```python
from build123d import *

# Parameters (mm, degrees)
BOSS_EXTRU_1_DEPTH      = 8
CONG_1_R                = 7.5
ENL_V_MAT_EXTRU_1_REACH = 29.299
ESQUISSE2_R             = 2
ESQUISSE3_R             = 7
ESQUISSE3_R_2           = 4
BOSS_EXTRU_2_DEPTH      = 8


with BuildPart() as part:
    # Esquisse1 → Boss.-Extru.1 (new body)
    with BuildSketch(Plane(origin=(0, 0, 0), x_dir=(1, 0, 0), z_dir=(0, 1, 0))):
        Polygon((0, -7.5), (25, -7.5), (25, 7.5), (0, 7.5), (-25, 7.5), (-25, -7.5), align=None)
    extrude(amount=BOSS_EXTRU_1_DEPTH)

    # Congé1
    cong_1_edges = [part.edges().sort_by_distance(p)[0] for p in [
        (-25, 4, 7.5),
        (-25, 4, -7.5),
        (25, 4, -7.5),
        (25, 4, 7.5),
    ]]
    fillet(cong_1_edges, radius=CONG_1_R - 0.0001)  # a hair under: the kernel refuses the full size

    # Esquisse2 → Enlèv. mat.-Extru.1 (cut, up to next)
    with BuildSketch(Plane(origin=(0, 8, 0), x_dir=(1, 0, 0), z_dir=(0, 1, 0)), mode=Mode.PRIVATE) as enl_v_mat_extru_1_sk1:
        with Locations(Location((-15, 0, 0), (0, 0, 270))):
            Circle(ESQUISSE2_R)
    enl_v_mat_extru_1_tool1 = extrude(enl_v_mat_extru_1_sk1.sketch, amount=-ENL_V_MAT_EXTRU_1_REACH, mode=Mode.PRIVATE) & part.part
    # Esquisse2 → Enlèv. mat.-Extru.1 (cut, up to next)
    with BuildSketch(Plane(origin=(0, 8, 0), x_dir=(1, 0, 0), z_dir=(0, 1, 0)), mode=Mode.PRIVATE) as enl_v_mat_extru_1_sk2:
        with Locations(Location((15, 0, 0), (0, 0, 270))):
            Circle(ESQUISSE2_R)
    enl_v_mat_extru_1_tool2 = extrude(enl_v_mat_extru_1_sk2.sketch, amount=-ENL_V_MAT_EXTRU_1_REACH, mode=Mode.PRIVATE) & part.part
    add(enl_v_mat_extru_1_tool1.solids().sort_by_distance((-15, 8, 0))[0], mode=Mode.SUBTRACT)
    add(enl_v_mat_extru_1_tool2.solids().sort_by_distance((15, 8, 0))[0], mode=Mode.SUBTRACT)

    # Esquisse3 → Boss.-Extru.2 (add)
    with BuildSketch(Plane(origin=(0, 8, 0), x_dir=(1, 0, 0), z_dir=(0, 1, 0))):
        with Locations(Location((0, 0, 0), (0, 0, 90))):
            Circle(ESQUISSE3_R)
        with Locations(Location((0, 0, 0), (0, 0, 270))):
            Circle(ESQUISSE3_R_2, mode=Mode.SUBTRACT)
    extrude(amount=BOSS_EXTRU_2_DEPTH)


solid = part.part
```
Could you check a few things on this model? Use its own coordinates, in mm. A direction names the side the tool comes from. Round coordinates to 2 decimals unless told otherwise and drop trailing zeros. Write each loop counter-clockwise with the first axis right and the second up, starting at its lowest first coordinate (ties: lowest second). Pieces come first, ordered by that corner, then holes. Notation, with made-up numbers: M 31,39 L 58,39 A27 ccw 58,62 Z; hole C -24.5,54.5 d8. An arc over 180 degrees is marked long. Answer in a Markdown table with one row per item. Add a question column.
Q1. Imagine slicing it at C-C (z = 1). Please give me the cut outline in (x, y), then the cut area to 3 significant figures.
Q2. Imagine slicing it at B-B (y = 2.25). Give the number of separate pieces and of enclosed holes in the cut face, then the cut area to 3 significant figures.
Q3. If I drill on line 1 (X direction, y = 4.25, z = 0); line 2 (X direction, y = 11.25, z = 0); line 3 (Y direction, x = -11, z = 4), over which ranges is the centre line in solid material (lowest first)? Write a range as from..to.
Q4. Imagine slicing it at A-A (x = 15). Please give me the cut outline in (y, z).
Q5. If we mould it in two halves opening along X, with no side actions, what happens to faces 1 (the cylindrical face through (-22.745, 4.056, -5.361)), 2 (the flat face through (0, 0, 0)), 3 (the cylindrical face through (-3.905, 11.944, -0.867)), 4 (the flat face through (0, 8, 0))? For each: +X half, -X half, draft (parallel to the pull), parting line (faces both ways), or undercut.
Q6. Imagine slicing it at D-D (x = 0). Please give me the cut outline in (y, z).
Q7. Will these pins go through, and if not, where does the flat tip stop? pin 1 Ø1.5 at (y, z) = (10.5, -6) entering from +X; pin 2 Ø5 at (y, z) = (8, -4) entering from +X; pin 3 Ø5 at (x, z) = (15, 0) entering from +Y; pin 4 Ø2 at (x, y) = (-9.5, 11) entering from +Z (3 decimals).
Q8. On a 3-axis mill with a long thin cutter (end or side, diameter ignored), from which of +Z, -Z, +X, -X, +Y, -Y can I reach the whole of each face in a straight line? I mean faces 5 (the flat face through (3, 16, -3)), 6 (the cylindrical face through (6.834, 11.944, 1.517)). Say none if no direction works.
Values:
| question | item | result |
|---|---|---|
| 1 | outline | M -24.93,0 L -16.73,0 L -16.73,8 L -24.93,8 Z; M -13.27,0 L 13.27,0 L 13.27,8 L 6.93,8 L 6.93,16 L 3.87,16 L 3.87,8 L -3.87,8 L -3.87,16 L -6.93,16 L -6.93,8 L -13.27,8 Z; M 16.73,0 L 24.93,0 L 24.93,8 L 16.73,8 Z |
| 1 | area | 392 mm^2 |
| 2 | separate pieces | 1 |
| 2 | enclosed holes | 2 |
| 2 | area | 677 mm^2 |
| 3 | line 1 | -25..-17, -13..13, 17..25 |
| 3 | line 2 | -7..-4, 4..7 |
| 3 | line 3 | 0..8 |
| 4 | outline | M 0,-7.5 L 8,-7.5 L 8,-2 L 0,-2 Z; M 0,2 L 8,2 L 8,7.5 L 0,7.5 Z |
| 5 | face 1 | -X half |
| 5 | face 2 | draft |
| 5 | face 3 | undercut |
| 5 | face 4 | undercut |
| 6 | outline | M 0,-7.5 L 8,-7.5 L 8,-7 L 16,-7 L 16,-4 L 8,-4 L 8,4 L 16,4 L 16,7 L 8,7 L 8,7.5 L 0,7.5 Z |
| 7 | pin 1 | x = 4.63 |
| 7 | pin 2 | x = 24.85 |
| 7 | pin 3 | y = 8 |
| 7 | pin 4 | through |
| 8 | face 5 | +Z, -Z, +X, -X, +Y |
| 8 | face 6 | +Y |
